Here's how the part is built. I have some questions about the finished solid (model axes, mm). Face numbers are marked on the shaded views. A direction names the side the tool comes from. Give positions to 0.01 mm unless a question says otherwise; leave off trailing zeros. Loops run counter-clockwise (first coordinate to the right, second up) from the corner with the lowest first, then second, coordinate; pieces in that order, holes last. Notation, with made-up numbers: (33.5, 87.5) - (83.5, 87.5) arc R26 ccw to (83.5, 123.5) - close; hole circle Ø7 at (35.5, 66). An arc over 180 degrees is marked (long way). One line per item, written item: value. Start each with the question number.
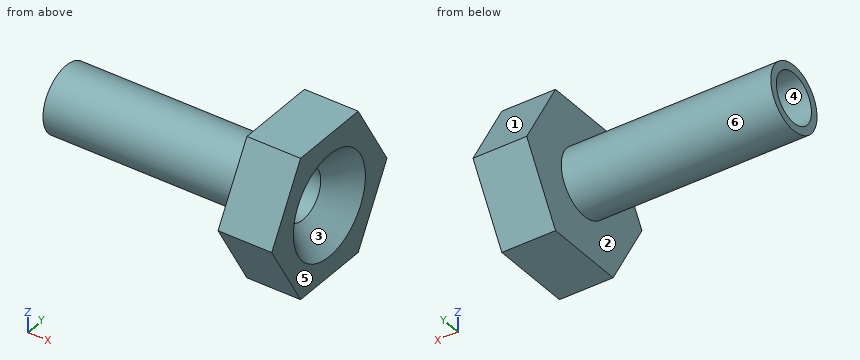
```python
from build123d import *

# Parameters (mm, degrees)
BOSS_EXTRUDE1_DEPTH = 2.05
SKETCH2_R           = 1.25
BOSS_EXTRUDE2_DEPTH = 8
SKETCH3_R           = 0.95
CUT_EXTRUDE1_DEPTH  = 11.863355835
CHAMFER1_SIZE       = 1


with BuildPart() as part:
    # Sketch1 → Boss-Extrude1 (new body)
    with BuildSketch(Plane(origin=(0, 0, 0), x_dir=(0, 0, -1), z_dir=(1, 0, 0))):
        Polygon((0, -3.117691454), (2.7, -1.558845727), (2.7, 1.558845727), (0, 3.117691454), (-2.7, 1.558845727), (-2.7, -1.558845727), align=None)
    extrude(amount=BOSS_EXTRUDE1_DEPTH)

    # Sketch2 → Boss-Extrude2 (add)
    with BuildSketch(Plane.ZY):
        with Locations(Location((0, 0, 0), (0, 0, 180))):
            Circle(SKETCH2_R)
    extrude(amount=BOSS_EXTRUDE2_DEPTH)

    # Sketch3 → Cut-Extrude1 (cut, through all)
    with BuildSketch(Plane.ZY.offset(8)):
        Circle(SKETCH3_R)
    extrude(amount=-CUT_EXTRUDE1_DEPTH, mode=Mode.SUBTRACT)

    # Chamfer1
    chamfer1_edges = [part.edges().sort_by_distance(p)[0] for p in [
        (2.05, 0, -0.95),
    ]]
    chamfer(chamfer1_edges, length=CHAMFER1_SIZE)


solid = part.part
```
(1) If we section it at A-A on y = 0: List the corners of the cut face in (x, z) for me.
(2) If we mould it in two halves opening along Y, with no side actions, what happens to the marked faces 3, 4, 5 and 6? For each: pulls with the +Y half, pulls with the -Y half, needs draft (parallel to the pull), parting line crosses it, or undercut.
(3) If we section it at B-B on x = -5: List the corners of the cut face in (y, z) for me.
(4) Will these pins go through, and if not, where does the flat tip stop? pin 1 (1 mm diameter, centred on x = -3.5, z = -0.5, fed in from +Y); pin 2 (1 mm diameter, centred on y = 1, z = 1.5, fed in from -X).
(5) Please list where these lines run through material, in increasing order: probe 1 along Y at (x, z) = (-4.75, 0); probe 2 along X at (y, z) = (2, 1.2); probe 3 along Z at (x, y) = (0.5, -0.75). Write a range as from..to.
(6) For the marked faces 1 and 2, which set-ups out of +Z, -Z, +X, -X, +Y, -Y let a thin tool reach every point of the face, with its end or its side?
(7) If we section it at C-C on z = -2.2: List the corners of the cut face in (x, y) for me.
Found:
1. outline: (-8, -1.25) - (0, -1.25) - (0, -2.7) - (2.05, -2.7) - (2.05, -1.95) - (1.05, -0.95) - (-8, -0.95) - close; (-8, 0.95) - (1.05, 0.95) - (2.05, 1.95) - (2.05, 2.7) - (0, 2.7) - (0, 1.25) - (-8, 1.25) - close
2. face 3: undercut
2. face 4: undercut
2. face 5: needs draft
2. face 6: parting line crosses it
3. outline: circle Ø2.5 at (0, 0); hole circle Ø1.9 at (0, 0)
4. pin 1: y = 1.25
4. pin 2: x = 0
5. probe 1: -1.25..-0.95, 0.95..1.25
5. probe 2: 0..2.05
5. probe 3: -2.7..-0.58, 0.58..2.7
6. face 1: +Z, +X, -X, +Y
6. face 2: -X
7. outline: (0, -1.85) - (2.05, -1.85) - (2.05, 1.85) - (0, 1.85) - close
